For this review, use the dimensioned drawing (mm, ordinates from the lowest corner) and the shaded views. A direction names the side the tool comes from. Coordinates: 2 decimals unless noted, no trailing zeros. Write each loop counter-clockwise with the first axis right and the second up, starting at its lowest first coordinate (ties: lowest second). Pieces come first, ordered by that corner, then holes. Notation, with made-up numbers: M 16.5,36.25 L 56.5,36.25 A18 cw 56.5,55.25 Z; hole C -21,70.25 d6. An arc over 180 degrees is marked long. One line per question, with ' | ' between items.
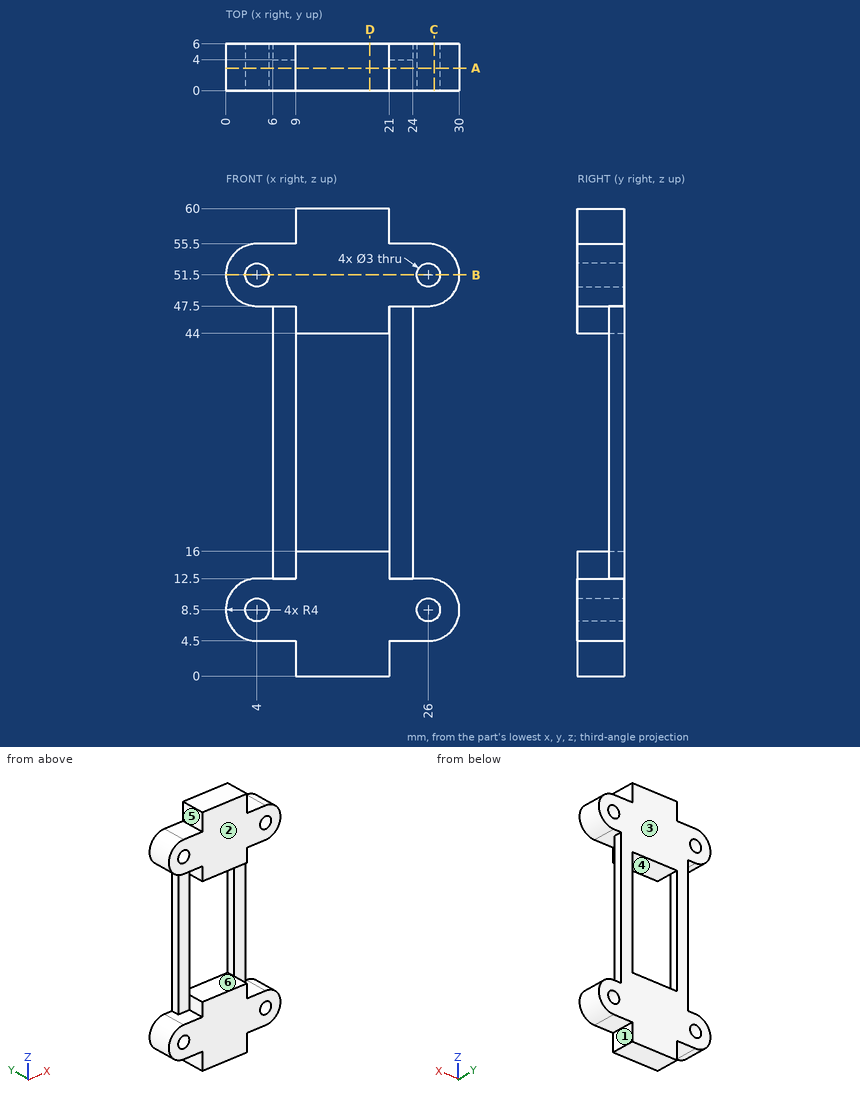
1) We need section B-B on z = 51.5. State the section outline as (x, y) points.
Responses:
outline: M 0,0 L 2.5,0 L 2.5,6 L 0,6 Z; M 5.5,0 L 24.5,0 L 24.5,6 L 5.5,6 Z; M 27.5,0 L 30,0 L 30,6 L 27.5,6 Z
2) Insertion check: pin 1 Ø3.5 at (x, z) = (4, 8.5) entering from -Y; pin 2 Ø1.8 at (y, z) = (2, 46.5) entering from -X; pin 3 Ø1.6 at (y, z) = (4.5, 26) entering from -X; pin 4 Ø1 at (y, z) = (5.5, 36) entering from +X. Each pin has a flat end and moves straight along its axis. Give the tip position at first contact, or say it passes through.
Responses:
pin 1: y = 0 | pin 2: x = 9 | pin 3: x = 6 | pin 4: x = 24
3) The part is to be moulded in two halves that separate along X. For the marked faces 3, 4, 5 and 6, say which applies: +X half, -X half, draft (parallel to the pull), parting line (faces both ways), or undercut.
Responses:
face 3: draft | face 4: undercut | face 5: -X half | face 6: undercut
4) We need section D-D on x = 18.5. State the section outline as (y, z) points, then the cut area to 3 significant figures.
Responses:
outline: M 0,0 L 6,0 L 6,16 L 0,16 Z; M 0,44 L 6,44 L 6,60 L 0,60 Z | area: 192 mm^2
5) Machinability: for the marked faces 1 and 2, which of the approach directions +Z, -Z, +X, -X, +Y, -Y give a long, thin tool a straight path to every point of the face, cutting with its end or side? Answer none if there is none.
Responses:
face 1: -Z, +X, +Y, -Y | face 2: +Z, -Z, +X, -X, -Y
6) We need section A-A on y = 2.9. State the section outline as (x, z) points.
Responses:
outline: M 4,4.5 L 9,4.5 L 9,0 L 21,0 L 21,4.5 L 26,4.5 A4 ccw 26,12.5 L 21,12.5 L 21,16 L 9,16 L 9,12.5 L 4,12.5 A4 ccw Z; M 4,47.5 L 9,47.5 L 9,44 L 21,44 L 21,47.5 L 26,47.5 A4 ccw 26,55.5 L 21,55.5 L 21,60 L 9,60 L 9,55.5 L 4,55.5 A4 ccw Z; hole C 4,8.5 d3; hole C 4,51.5 d3; hole C 26,8.5 d3; hole C 26,51.5 d3
7) To check wall thickness, follow line 1 along X through (y, z) = (2.2, 51.5); line 2 along X through (y, z) = (5.15, 34); line 3 along Z through (x, y) = (20.75, 5.4). State the ranges of each line that lie inside material, in increasing order. Write a range as [from, to].
Responses:
line 1: [0, 2.5], [5.5, 24.5], [27.5, 30] | line 2: [6, 9], [21, 24] | line 3: [0, 16], [44, 60]
8) We need section C-C on x = 26.75. State the section outline as (y, z) points, then the cut area to 3 significant figures.
Responses:
outline: M 0,4.57 L 6,4.57 L 6,7.2 L 0,7.2 Z; M 0,9.8 L 6,9.8 L 6,12.43 L 0,12.43 Z; M 0,47.57 L 6,47.57 L 6,50.2 L 0,50.2 Z; M 0,52.8 L 6,52.8 L 6,55.43 L 0,55.43 Z | area: 63.1 mm^2
